Drawing for the job (mm, zero at the part's lowest x, y, z). Coordinates: 2 decimals unless noted, no trailing zeros. Write each loop counter-clockwise with the first axis right and the second up, starting at its lowest first coordinate (ties: lowest second). Pieces come first, ordered by that corner, then holes. Notation, with made-up numbers: M 86,-33 L 100,-33 A16 cw 100,-9 Z; hole C -34.5,-14.75 d2. An arc over 180 degrees is marked long. Put each result on its own line as item: value. Start each with the question number.
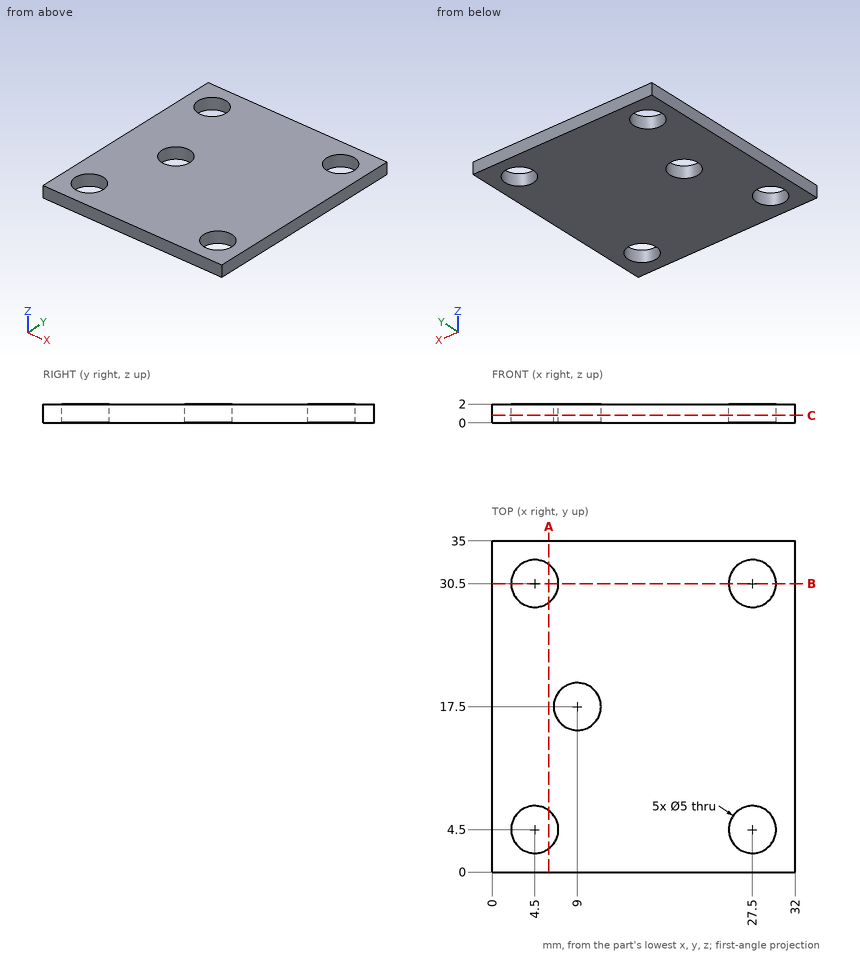
(1) Slice it at A-A, the plane x = 6. Write the cut outline in (y, z), then the cut area to 3 significant figures.
(2) Drill centre lines: line 1 (Y direction, x = 4.5, z = 1.15); line 2 (Y direction, x = 9, z = 0.55); line 3 (X direction, y = 3, z = 1.55). Where is each one in solid material? Low to high. Write a range as [from, to].
(3) Slice it at C-C, the plane z = 0.8. Write the cut outline in (x, y), then the cut area to 3 significant figures.
(4) Slice it at B-B, the plane y = 30.5. Write the cut outline in (x, z), then the cut area to 3 significant figures.
Result set:
1. outline: M 0,0 L 2.5,0 L 2.5,2 L 0,2 Z; M 6.5,0 L 28.5,0 L 28.5,2 L 6.5,2 Z; M 32.5,0 L 35,0 L 35,2 L 32.5,2 Z
1. area: 54.0 mm^2
2. line 1: y = [0, 2], [7, 28], [33, 35]
2. line 2: y = [0, 15], [20, 35]
2. line 3: x = [0, 2.5], [6.5, 25.5], [29.5, 32]
3. outline: M 0,0 L 32,0 L 32,35 L 0,35 Z; hole C 4.5,4.5 d5; hole C 4.5,30.5 d5; hole C 9,17.5 d5; hole C 27.5,4.5 d5; hole C 27.5,30.5 d5
3. area: 1,020 mm^2
4. outline: M 0,0 L 2,0 L 2,2 L 0,2 Z; M 7,0 L 25,0 L 25,2 L 7,2 Z; M 30,0 L 32,0 L 32,2 L 30,2 Z
4. area: 44.0 mm^2
